Input: dimensioned drawing with shaded views. Units: mm. Origin: part minimum x, y, z. Coordinates: 2 decimals unless noted, no trailing zeros. Order: outer loops, then holes, each group sorted by start corner. A loop starts at its lowest first (then second) coordinate and runs counter-clockwise, first axis right, second up.
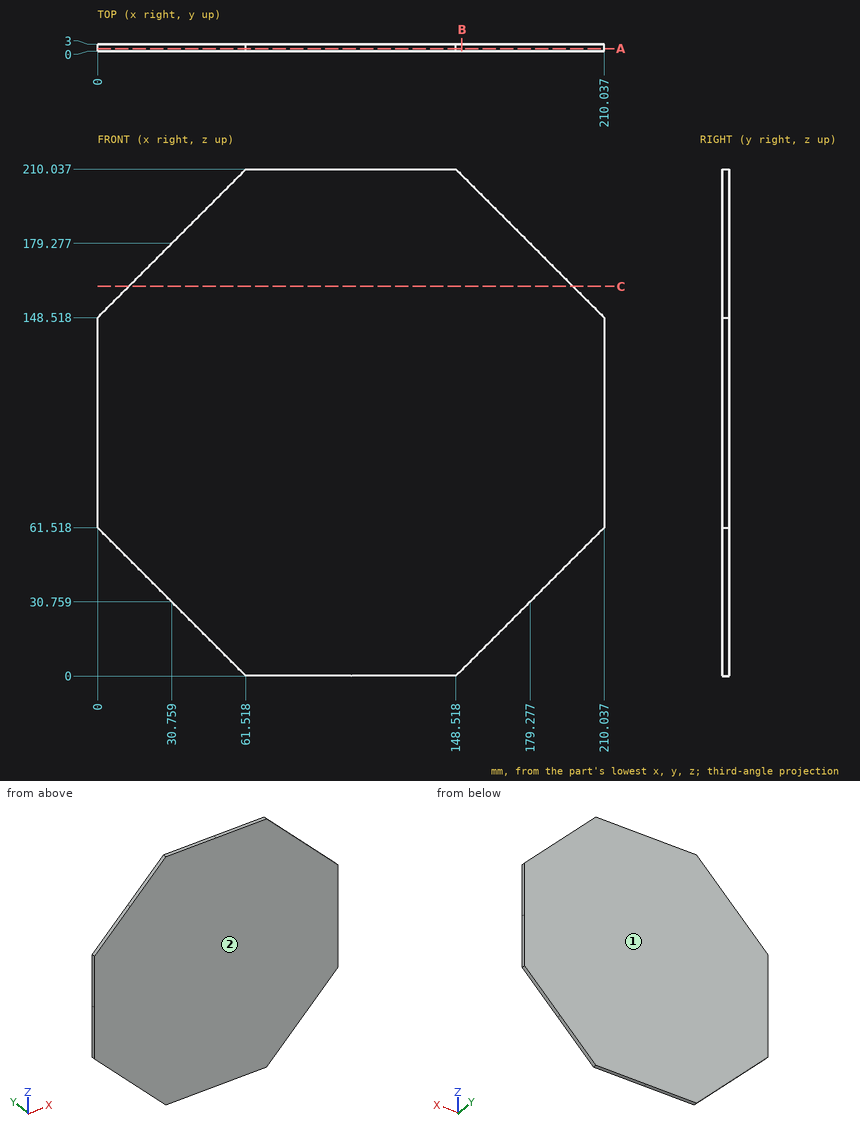
1. Ray query, line 1 (Z direction, x = 49, y = 1.75); line 2 (Z direction, x = 167.5, y = 0.5) (1 decimal); line 3 (X direction, y = 1.7, z = 34.5). Return the intervals inside material, ascending.
Findings:
line 1: z = 12.52 to 197.52
line 2: z = 19 to 191.1
line 3: x = 27.02 to 183.02
2. Pin query (flat end, axial travel): P1, Ø1.5, axis at y = 2, z = 55.5, coming from the -X side; P2, Ø1.5, axis at x = 53.5, y = 1.5, coming from the +Z side. Return the tip coordinate at first contact, or that it passes through.
Findings:
P1: stops at x = 5.27
P2: stops at z = 202.77
3. Section query A-A on y = 1.1. Return loops of the section in (x, z), plus the area to 3 significant figures.
Findings:
outline: (0, 61.52) - (61.52, 0) - (148.52, 0) - (210.04, 61.52) - (210.04, 148.52) - (148.52, 210.04) - (61.52, 210.04) - (0, 148.52) - close
area: 36,500 mm2
4. Section query B-B on x = 151. Return loops of the section in (y, z) (1 decimal).
Findings:
outline: (0, 2.5) - (3, 2.5) - (3, 207.6) - (0, 207.6) - close
5. Draft query along Y for the marked faces 1 and 2. Return one class per face: released by +Y, released by -Y, zero draft, split by the parting line, or undercut.
Findings:
face 1: released by +Y
face 2: released by -Y
6. Section query C-C on z = 161.5. Return loops of the section in (x, y) (1 decimal).
Findings:
outline: (13, 0) - (197.1, 0) - (197.1, 3) - (13, 3) - close
